from build123d import *

# Parameters (mm, degrees)
CROQUIS1_W               = 34
CROQUIS1_H               = 24
SALIENTE_EXTRUIR1_DEPTH  = 3
CROQUIS2_W               = 30
CROQUIS2_H               = 20
CORTAR_EXTRUIR1_DEPTH    = 1
CROQUIS6_R               = 1.5
SALIENTE_EXTRUIR3_DEPTH  = 1.5
MATRIZL1_COUNT           = 2
MATRIZL1_PITCH           = 23
CROQUIS8_W               = 5
CROQUIS8_H               = 0.71
SALIENTE_EXTRUIR5_DEPTH  = 0.2
CROQUIS10_W              = 5
CROQUIS10_H              = 0.71
SALIENTE_EXTRUIR6_DEPTH  = 0.2
CROQUIS18_W              = 15
CROQUIS18_H              = 3.5
SALIENTE_EXTRUIR8_DEPTH  = 0.2
CROQUIS23_W              = 34
CROQUIS23_H              = 24
SALIENTE_EXTRUIR11_DEPTH = 2


with BuildPart() as part:
    # Croquis1 → Saliente-Extruir1 (new body)
    with BuildSketch(Plane(origin=(0, 0, 0), x_dir=(1, 0, 0), z_dir=(0, 1, 0))):
        Rectangle(CROQUIS1_W, CROQUIS1_H)
    extrude(amount=SALIENTE_EXTRUIR1_DEPTH)

    # Croquis2 → Cortar-Extruir1 (cut)
    with BuildSketch(Plane(origin=(0, 3, 0), x_dir=(1, 0, 0), z_dir=(0, 1, 0))):
        Rectangle(CROQUIS2_W, CROQUIS2_H)
    extrude(amount=-CORTAR_EXTRUIR1_DEPTH, mode=Mode.SUBTRACT)

    # Croquis6 → Saliente-Extruir3 (add)
    with BuildSketch(Plane(origin=(-1.755264317, 2, -0.109917309), x_dir=(1, 0, 0), z_dir=(0, 1, 0))):
        with Locations(Location((-9.854739848, -0.135008356, 0), (0, 0, 270))):
            Circle(CROQUIS6_R)
    saliente_extruir3 = extrude(amount=SALIENTE_EXTRUIR3_DEPTH)

    # MatrizL1: Saliente-Extruir3 ×2
    with Locations(*[(i * MATRIZL1_PITCH, 0, 0) for i in range(1, MATRIZL1_COUNT)]):
        add(saliente_extruir3)

    # Croquis8 → Saliente-Extruir5 (add)
    with BuildSketch(Plane(origin=(0, 2, 0.512947444), x_dir=(1, 0, 0), z_dir=(0, 1, 0))):
        with Locations((-9.175591951, 0.49731844)):
            Rectangle(CROQUIS8_W, CROQUIS8_H)
    extrude(amount=SALIENTE_EXTRUIR5_DEPTH)

    # Croquis10 → Saliente-Extruir6 (add)
    with BuildSketch(Plane(origin=(3.639202125, 2, -0.512947444), x_dir=(1, 0, 0), z_dir=(0, 1, 0))):
        with Locations((5.490278272, -0.538512576)):
            Rectangle(CROQUIS10_W, CROQUIS10_H)
    extrude(amount=SALIENTE_EXTRUIR6_DEPTH)

    # Croquis18 → Saliente-Extruir8 (add)
    with BuildSketch(Plane(origin=(0, 2, 0), x_dir=(1, 0, 0), z_dir=(0, 1, 0))):
        Rectangle(CROQUIS18_W, CROQUIS18_H)
    extrude(amount=SALIENTE_EXTRUIR8_DEPTH)

    # Croquis23 → Saliente-Extruir11 (add)
    with BuildSketch(Plane.XZ):
        Rectangle(CROQUIS23_W, CROQUIS23_H)
    extrude(amount=SALIENTE_EXTRUIR11_DEPTH)


solid = part.part
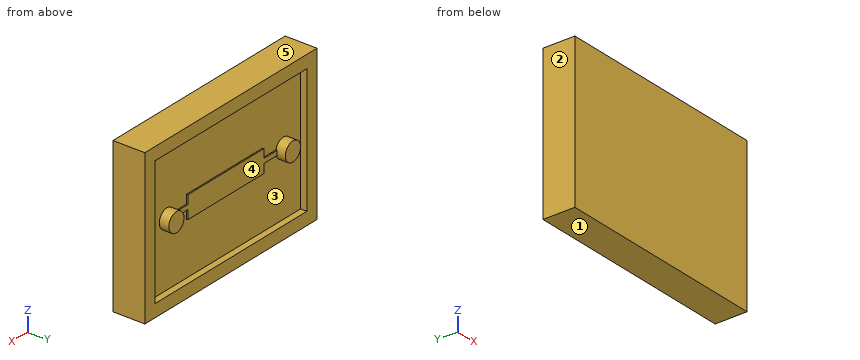
CAD build for the part. Positions are in the model's coordinates, mm. Face numbers are marked on the shaded views. A direction names the side the tool comes from. Round coordinates to 2 decimals unless told otherwise and drop trailing zeros. Loops run counter-clockwise (first coordinate to the right, second up) from the corner with the lowest first, then second, coordinate; pieces in that order, holes last. Notation, with made-up numbers: (67, 71.5) - (98, 71.5) arc R6 cw to (98, 76.5) - close; hole circle Ø1 at (85, -20.5). An arc over 180 degrees is marked (long way). Put each result on its own line as item: value.
1. 3-axis set-ups, long thin cutter, end or side, ignore diameter. For the marked faces 4 and 5: which of +Z, -Z, +X, -X, +Y, -Y reach the whole face in a straight line?
Geometry check:
face 4: +Y
face 5: +Z, +X, -X, +Y, -Y
2. Two-plate mould, pull along Z, no slides. Class the marked faces 1, 2 and 3: released by +Z, released by -Z, zero draft, split by the parting line, or undercut.
Geometry check:
face 1: released by -Z
face 2: zero draft
face 3: undercut
3. Pin check, flat tips, straight feed: P1, Ø12, axis at x = -12.5, z = -6, coming from the +Y side; P2, Ø12, axis at x = 8, z = 8, coming from the +Y side; P3, Ø4, axis at x = 4.5, z = 0, coming from the +Y side. Stop position of each tip, or through.
Geometry check:
P1: y = 3.5
P2: y = 3
P3: y = 2.2
4. Slice it at C-C on x = 4. List the corners of the cut face in (y, z), and give its area (3 significant figures).
Geometry check:
outline: (-2, -12) - (3, -12) - (3, -10) - (2, -10) - (2, -1.75) - (2.2, -1.75) - (2.2, 1.75) - (2, 1.75) - (2, 10) - (3, 10) - (3, 12) - (-2, 12) - close
area: 101 mm²
5. Slice it at A-A on z = 7.75. List the corners of the cut face in (x, y).
Geometry check:
outline: (-17, -2) - (17, -2) - (17, 3) - (15, 3) - (15, 2) - (-15, 2) - (-15, 3) - (-17, 3) - close
6. Wall check: line 1 (Z direction, x = 7, y = 2.65); line 2 (Y direction, x = 12.5, z = -3); line 3 (Y direction, x = 3.5, z = 1.5). Give the ranges that are in metal, low to high.
Geometry check:
line 1: -12 to -10, 10 to 12
line 2: -2 to 2
line 3: -2 to 2.2
7. Slice it at B-B on x = -8.5. List the corners of the cut face in (y, z).
Geometry check:
outline: (-2, -12) - (3, -12) - (3, -10) - (2, -10) - (2, -0.34) - (2.2, -0.34) - (2.2, 0.37) - (2, 0.37) - (2, 10) - (3, 10) - (3, 12) - (-2, 12) - close
8. Slice it at D-D on z = 1. List the corners of the cut face in (x, y), and give its area (3 significant figures).
Geometry check:
outline: (-17, -2) - (17, -2) - (17, 3) - (15, 3) - (15, 2) - (12.53, 2) - (12.53, 3.5) - (10.25, 3.5) - (10.25, 2) - (7.5, 2) - (7.5, 2.2) - (-7.5, 2.2) - (-7.5, 2) - (-10.47, 2) - (-10.47, 3.5) - (-12.75, 3.5) - (-12.75, 2) - (-15, 2) - (-15, 3) - (-17, 3) - close
area: 150 mm²
